```python
from build123d import *

# Parameters (mm, degrees)
SKETCH1_R           = 160
SKETCH1_R_2         = 80
SKETCH1_R_3         = 9.25
BOSS_EXTRUDE1_DEPTH = 6


with BuildPart() as part:
    # Sketch1 → Boss-Extrude1 (new, symmetric)
    with BuildSketch(Plane.XY):
        Circle(SKETCH1_R)
        Circle(SKETCH1_R_2, mode=Mode.SUBTRACT)
        with Locations((-96.844081606, 101.100068535)):
            Circle(SKETCH1_R_3, mode=Mode.SUBTRACT)
        with Locations((3.009437218, 139.967650861)):
            Circle(SKETCH1_R_3, mode=Mode.SUBTRACT)
        with Locations((101.100068535, 96.844081606)):
            Circle(SKETCH1_R_3, mode=Mode.SUBTRACT)
        with Locations((139.967650861, -3.009437218)):
            Circle(SKETCH1_R_3, mode=Mode.SUBTRACT)
        with Locations((96.844081606, -101.100068535)):
            Circle(SKETCH1_R_3, mode=Mode.SUBTRACT)
        with Locations((-3.009437218, -139.967650861)):
            Circle(SKETCH1_R_3, mode=Mode.SUBTRACT)
        with Locations((-101.100068535, -96.844081606)):
            Circle(SKETCH1_R_3, mode=Mode.SUBTRACT)
        with Locations((-139.967650861, 3.009437218)):
            Circle(SKETCH1_R_3, mode=Mode.SUBTRACT)
    extrude(amount=BOSS_EXTRUDE1_DEPTH, both=True)


solid = part.part
```
Geometry: final body of the model. Coordinates: model frame, mm. Round coordinates to 2 decimals unless told otherwise and drop trailing zeros. Write each loop counter-clockwise with the first axis right and the second up, starting at its lowest first coordinate (ties: lowest second). Pieces come first, ordered by that corner, then holes. Notation, with made-up numbers: (83, 2.25) -> (87, 2.25) arc R27 ccw to (87, 28.25) -> close; hole circle Ø2 at (81.5, 48.5). An arc over 180 degrees is marked (long way). Use CSV: the item, a comma, the result in double quotes. Start each with the question number.
Q1. Pull-direction query (Y, two-part tool) for faces 1 (the face through (-73.4, -33.3, 6)), 2 (the face through (-96.83, -105.05, -0.08)), 3 (the face through (-34.685, -156.195, 0.084)); classes: pulls with the +Y half, pulls with the -Y half, needs draft (parallel to the pull), parting line crosses it, or undercut.
Q2. First-contact query: pin 1 Ø21.5 at (x, y) = (101.1, 96.84) entering from +Z; pin 2 Ø5 at (x, z) = (-108, 2.5) entering from +Y; pin 3 Ø1 at (x, z) = (109, -2.5) entering from -Y; pin 4 Ø2 at (y, z) = (-91.5, -4) entering from -X. Flat tips, straight axial feed; report the tip coordinate or a pass-through.
Q3. Section A-A (x = -37). Return loops of the section in (y, z), plus the area to 3 significant figures.
Q4. Section B-B (x = 0). Return loops of the section in (y, z).
Q5. Section D-D (y = 126.5). Return loops of the section in (x, z).
Q6. Section C-C (z = -4). Give the number of separate pieces and of enclosed holes in the cut face, plus the area to 3 significant figures.
Q7. Line query: L1, parallel to Y at x = 93, z = 2; L2, parallel to Y at x = -95.5, z = 2.5; L3, parallel to X at y = -11, z = 3.5. Output: solid intervals per line, ascending.
Result sheet:
1,face 1,"needs draft"
1,face 2,"undercut"
1,face 3,"parting line crosses it"
2,pin 1,"z = 6"
2,pin 2,"y = 120.29"
2,pin 3,"y = -117.59"
2,pin 4,"x = -131.95"
3,outline,"(-155.66, -6) -> (-70.93, -6) -> (-70.93, 6) -> (-155.66, 6) -> close; (70.93, -6) -> (155.66, -6) -> (155.66, 6) -> (70.93, 6) -> close"
3,area,"2,030 mm²"
4,outline,"(-160, -6) -> (-148.71, -6) -> (-148.71, 6) -> (-160, 6) -> close; (-131.22, -6) -> (-80, -6) -> (-80, 6) -> (-131.22, 6) -> close; (80, -6) -> (131.22, -6) -> (131.22, 6) -> (80, 6) -> close; (148.71, -6) -> (160, -6) -> (160, 6) -> (148.71, 6) -> close"
5,outline,"(-97.97, -6) -> (97.97, -6) -> (97.97, 6) -> (-97.97, 6) -> close"
6,separate pieces,"1"
6,enclosed holes,"9"
6,area,"58,200 mm²"
7,L1,"-130.2 to -109.51, -92.69 to 92.38, 101.31 to 130.2"
7,L2,"-128.37 to -104.21, -89.48 to 91.95, 110.25 to 128.37"
7,L3,"-159.62 to -79.24, 79.24 to 135.31, 144.63 to 159.62"
